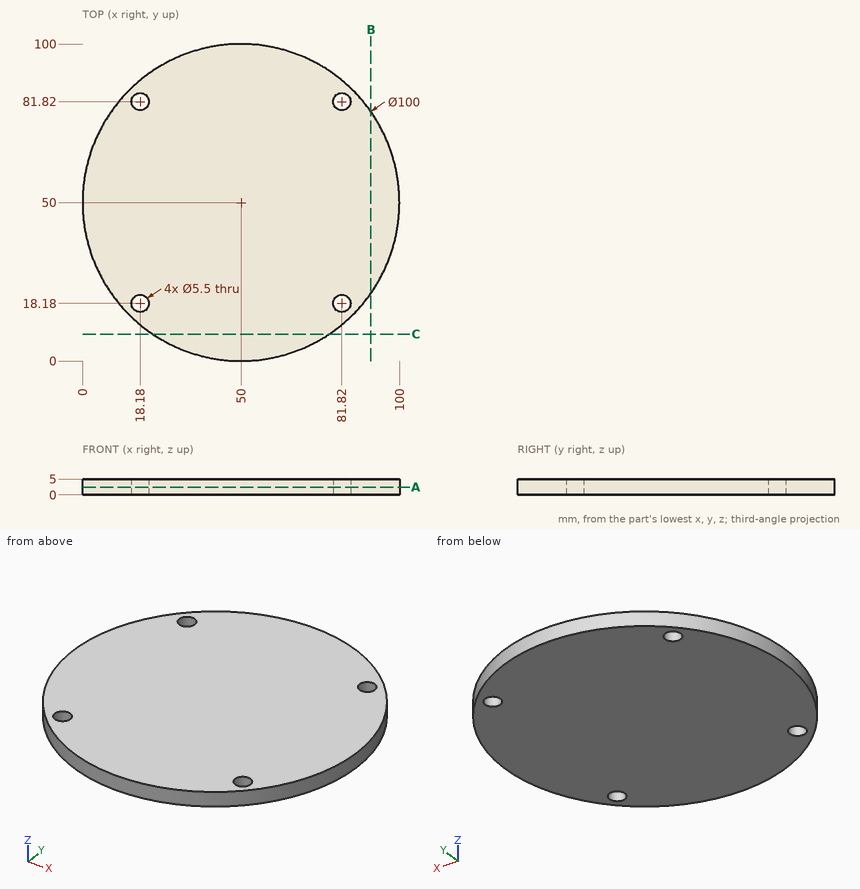
Here's the drawing with two shaded views (mm, measured from the low corner). I have some questions. Round coordinates to 2 decimals unless told otherwise and drop trailing zeros. Order: outer loops, then holes, each group sorted by start corner. A loop starts at its lowest first (then second) coordinate and runs counter-clockwise, first axis right, second up. Notation, with made-up numbers: (65.25, 84) -> (77.25, 84) arc R19 ccw to (77.25, 113) -> close; hole circle Ø5 at (56.5, 75). An arc over 180 degrees is marked (long way). Use a Markdown table: item, result. Add a question column.
(1) Suppose I cut it at A-A, the plane z = 2.45. Please give me the cut outline in (x, y).
(2) Suppose I cut it at B-B, the plane x = 91. Please give me the cut outline in (y, z).
(3) Suppose I cut it at C-C, the plane y = 8.5. Please give me the cut outline in (x, z).
(4) I need wall thicknesses on line 1 along Y through (x, z) = (16.5, 3.6); line 2 along X through (y, z) = (82, 0.75) (1 decimal); line 3 along Y through (x, z) = (19.5, 0.35). Which ranges of each line are inside material? Lowest first, please.
(5) For pin 1 Ø3 at (x, z) = (63, 1.5) entering from +Y; pin 2 Ø1 at (y, z) = (37.5, 2) entering from +X, each with a flat end and sliding along its axis, tell me the tip position at first contact or that it passes through.
Verdict:
| question | item | result |
|---|---|---|
| 1 | outline | circle Ø100 at (50, 50); hole circle Ø5.5 at (18.18, 18.18); hole circle Ø5.5 at (18.18, 81.82); hole circle Ø5.5 at (81.82, 18.18); hole circle Ø5.5 at (81.82, 81.82) |
| 2 | outline | (21.38, 0) -> (78.62, 0) -> (78.62, 5) -> (21.38, 5) -> close |
| 3 | outline | (22.11, 0) -> (77.89, 0) -> (77.89, 5) -> (22.11, 5) -> close |
| 4 | line 1 | 12.88 to 16, 20.36 to 79.64, 84 to 87.12 |
| 4 | line 2 | 11.6 to 15.4, 20.9 to 79.1, 84.6 to 88.4 |
| 4 | line 3 | 10.38 to 15.77, 20.59 to 79.41, 84.23 to 89.62 |
| 5 | pin 1 | y = 98.66 |
| 5 | pin 2 | x = 98.54 |
